```python
from build123d import *

# Parameters (mm, degrees)
SKETCH2_R   = 13
SKETCH2_R_2 = 10


with BuildPart() as part:
    # Sweep-Thin1: sweep along a path in Sketch1
    with BuildLine(Plane(origin=(0, 0, 0), x_dir=(0, 0, -1), z_dir=(1, 0, 0))) as sweep_thin1_path:
        Line((0, 33.456749572), (-20, 33.456749572))
        ThreePointArc((-20, 33.456749572), (-41.213203436, 24.669953007), (-50, 3.456749572))
        Line((-50, 3.456749572), (-50, -76.543250428))
    # Sketch2 → Sweep-Thin1 (sweep)
    with BuildSketch(Plane.XY):
        with Locations((0, 33.456749572)):
            Circle(SKETCH2_R)
        with Locations((0, 33.456749572)):
            Circle(SKETCH2_R_2, mode=Mode.SUBTRACT)
    sweep(path=sweep_thin1_path.line)


solid = part.part
```
The model under review builds one solid part; all positions refer to its coordinate system, in mm. A direction names the side the tool comes from. Round coordinates to 2 decimals unless told otherwise and drop trailing zeros. Write each loop counter-clockwise with the first axis right and the second up, starting at its lowest first coordinate (ties: lowest second). Pieces come first, ordered by that corner, then holes. Notation, with made-up numbers: (-31.75, -24) - (-12.75, -24) arc R14 cw to (-12.75, -8) - close; hole circle Ø8 at (73, 19.5). An arc over 180 degrees is marked (long way). Answer as CSV lines item,"result". Start each with the question number.
(1) We need section C-C on z = 12.5. State the section outline as (x, y) points, plus the area to 3 significant figures.
(2) We need section A-A on x = 0. State the section outline as (y, z) points.
(3) We need section B-B on y = -48. State the section outline as (x, z) points, plus the area to 3 significant figures.
(4) For pin 1 Ø12 at (x, y) = (0, 33.46) entering from -Z; pin 2 Ø4 at (x, y) = (10.5, 4) entering from +Z; pin 3 Ø1 at (x, y) = (-4, -42.5) entering from +Z, all flat-tipped, find the tip position at first contact; note any pin that passes through.
(5) Draft analysis for pull direction X (two halves, no side actions). For faces 1 (the cylindrical face through (-9.582, 42.243, 10.14)), 2 (the cylindrical face through (-1.3, 43.37, 10.14)), 3 (the flat face through (7, 26, 0)), state which applies: pulls with the +X half, pulls with the -X half, needs draft (parallel to the pull), parting line crosses it, or undercut.
(6) For faces 4 (the flat face through (-8, -76.543, 43)), 5 (the cylindrical face through (-1.69, -37.1, 62.89)), list the 3-axis set-ups (+Z, -Z, +X, -X, +Y, -Y) from which the entire face can be reached by the end or side of a thin tool; tool diameter is ignored.
(7) To check wall thickness, follow line 1 (X direction, y = -34, z = 50); line 2 (Y direction, x = 0, z = 7); line 3 (Z direction, x = 0, y = -38.5). State the ranges of each line that lie inside material, in increasing order.
Worked answers:
1,outline,"circle Ø26 at (0, 33.46); hole circle Ø20 at (0, 33.46)"
1,area,"217 mm²"
2,outline,"(-76.54, 37) - (3.46, 37) arc R17 cw to (20.46, 20) - (20.46, 0) - (23.46, 0) - (23.46, 20) arc R20 ccw to (3.46, 40) - (-76.54, 40) - close; (-76.54, 60) - (3.46, 60) arc R40 cw to (43.46, 20) - (43.46, 0) - (46.46, 0) - (46.46, 20) arc R43 ccw to (3.46, 63) - (-76.54, 63) - close"
3,outline,"circle Ø26 at (0, 50); hole circle Ø20 at (0, 50)"
3,area,"217 mm²"
4,pin 1,"z = 37.43"
4,pin 2,"z = 59.83"
4,pin 3,"z = 62.52"
5,face 1,"parting line crosses it"
5,face 2,"undercut"
5,face 3,"needs draft"
6,face 4,"+Z, -Z, +X, -X, -Y"
6,face 5,"-Y"
7,line 1,"-13 to -10, 10 to 13"
7,line 2,"20.46 to 23.46, 43.46 to 46.46"
7,line 3,"37 to 40, 60 to 63"
